from build123d import *

# Parameters (mm, degrees)
F0_R     = 2
F1_DEPTH = 10
F2_R     = 1
F3_W     = 15
F3_H     = 7
F4_DEPTH = 6
F5_R     = 2.5
F6_R     = 2
F7_DEPTH = 25.4


with BuildPart() as f1:
    # F0 (on Right) → F1 (new body)
    with BuildSketch(Plane.YZ):
        Polygon((0, 51), (0, 0), (6, 0), (6, 17), (27, 17), (27, 0), (33, 0), (33, 51), align=None)
        with Locations((16.199438, 23)):
            Circle(F0_R, mode=Mode.SUBTRACT)
    extrude(amount=-F1_DEPTH)

    # F2
    f2_edges = [f1.edges().sort_by_distance(p)[0] for p in [
        (-10, 16.5, 51),
    ]]
    fillet(f2_edges, radius=F2_R)

    # F3 (on face) → F4 (join)
    with BuildSketch(Plane(origin=(-10, 0, 0), x_dir=(0, -1, 0), z_dir=(-1, 0, 0))):
        with Locations((-16.5, 32.5)):
            Rectangle(F3_W, F3_H)
    extrude(amount=F4_DEPTH)

    # F5
    f5_edges = [f1.edges().sort_by_distance(p)[0] for p in [
        (-16, 16.5, 36),
        (-16, 16.5, 29),
    ]]
    fillet(f5_edges, radius=F5_R)

    # F6 (on face) → F7 (cut)
    with BuildSketch(Plane(origin=(0, 24, 0), x_dir=(-1, 0, 0), z_dir=(0, 1, 0))):
        with Locations((12.673163, 32.804124)):
            Circle(F6_R)
    extrude(amount=-F7_DEPTH, mode=Mode.SUBTRACT)


solid = f1.part
Design review of the part built by this model. Coordinates are the model's own, in mm. A direction names the side the tool comes from. Round coordinates to 2 decimals unless told otherwise and drop trailing zeros. Write each loop counter-clockwise with the first axis right and the second up, starting at its lowest first coordinate (ties: lowest second). Pieces come first, ordered by that corner, then holes. Notation, with made-up numbers: (-20, 67.25) - (27, 67.25) arc R10 ccw to (27, 77.25) - close; hole circle Ø10 at (43, 83). An arc over 180 degrees is marked (long way). Return JSON: item names as keys, results as strings. Group by question number.
Item 1: We need section B-B on y = 3.5. Write out the cut boundary in (x, z), and give its area (3 significant figures).
Item 2: We need section C-C on x = -11.5. Write out the cut boundary in (y, z), and give its area (3 significant figures).
Item 3: We need section D-D on y = 11. Write out the cut boundary in (x, z), and give its area (3 significant figures).
Item 4: Insertion check: P1, Ø1, axis at y = 17.5, z = 29.5, coming from the -X side; P2, Ø1.5, axis at x = -13.5, y = 22.5, coming from the +Z side; P3, Ø1, axis at x = -11.5, y = 17, coming from the -Z side; P4, Ø3.5, axis at y = 16.2, z = 23, coming from the -X side. Each pin has a flat end and moves straight along its axis. Give the tip position at first contact, or say it passes through.
Item 5: The part is to be moulded in two halves that separate along Y. For faces 1 (the face through (-15.248, 16.395, 35.287)), 2 (the face through (-14, 9, 31)), 3 (the face through (-4.93, 18.047, 22.234)), say which applies: pulls with the +Y half, pulls with the -Y half, needs draft (parallel to the pull), parting line crosses it, or undercut.
Item 6: For probe 1 along Y at (x, z) = (-1, 7); probe 2 along Z at (x, y) = (-3.75, 12); probe 3 along X at (y, z) = (18.5, 23), list the stretches that pass through material, from the lowest coordinate up. Write a range as [from, to].
Item 7: Machinability: for faces 4 (the face through (-5, 16, 17)), 5 (the face through (-4, 17, 51)), 6 (the face through (-12, 17, 29)), 7 (the face through (-12, 17, 36)), which of the approach directions +Z, -Z, +X, -X, +Y, -Y give a long, thin tool a straight path to every point of the face, cutting with its end or side? Answer none if there is none.
Item 8: We need section A-A on z = 15.5. Write out the cut boundary in (x, y).
Model answer:
{
 "1": {"outline": "(-10, 0) - (0, 0) - (0, 51) - (-9, 51) arc R1 ccw to (-10, 50) - close", "area": "510 mm²"},
 "2": {"outline": "(9, 29) - (24, 29) - (24, 31.18) - (9, 31.18) - close; (9, 34.42) - (24, 34.42) - (24, 36) - (9, 36) - close", "area": "56.4 mm²"},
 "3": {"outline": "(-16, 31.5) arc R2.5 ccw to (-13.5, 29) - (-10, 29) - (-10, 17) - (0, 17) - (0, 51) - (-9, 51) arc R1 ccw to (-10, 50) - (-10, 36) - (-13.5, 36) arc R2.5 ccw to (-16, 33.5) - close; hole circle Ø4 at (-12.67, 32.8)", "area": "367 mm²"},
 "4": {"P1": "stops at x = -15.5", "P2": "stops at z = 36", "P3": "stops at z = 29", "P4": "passes through"},
 "5": {"face 1": "needs draft", "face 2": "pulls with the -Y half", "face 3": "undercut"},
 "6": {"probe 1": "y = [0, 6], [27, 33]", "probe 2": "z = [17, 51]", "probe 3": "x = [-10, 0]"},
 "7": {"face 4": "-Z, +X, -X", "face 5": "+Z, +X, -X, +Y, -Y", "face 6": "-Z, -X, +Y, -Y", "face 7": "+Z, -X, +Y, -Y"},
 "8": {"outline": "(-10, 0) - (0, 0) - (0, 6) - (-10, 6) - close; (-10, 27) - (0, 27) - (0, 33) - (-10, 33) - close"}
}
